Autodesk Inventor part; units mm, degrees
ref_plane "YZ Plane" through (0, 0, 0) normal (1, 0, 0) x (0, 1, 0)
ref_plane "XZ Plane" through (0, 0, 0) normal (0, 1, 0) x (-1, 0, 0)
ref_plane "XY Plane" through (0, 0, 0) normal (0, 0, 1) x (1, 0, 0)
sketch "Sketch_1" plane through (0, 0, 0) normal (0, 0, 1) x (1, 0, 0)
  line L0 (23, 0) -> (0, 0)
  line L1 (0, 0) -> (0, 4.5)
  line L2 (0, 4.5) -> (0.5, 5)
  line L3 (0.5, 5) -> (22.5, 5)
  line L4 (22.5, 5) -> (23, 4.5)
  line L5 (23, 4.5) -> (23, 0)
  line L6 (23, 0) -> (0, 0)
revolve "Revolution1" add sketch "Sketch_1" angle 360 about axis through (23, 0, 0) along (1, 0, 0)
sketch "Sketch2" plane through (0, 0, 0) normal (-1, 0, 0) x (0, 0, 1)
  point P0 (0, 0)
hole "Hole1" at (0, 0, 0) direction (1, 0, 0) diameter 4.134 depth 15.3066 tip angle 120 countersink diameter 5 countersink angle 90
sketch "Sketch_8" plane through (0, 0, 0) normal (0, 0, 1) x (1, 0, 0)
  line L0 (23, 0) -> (-23, 0)
  line L1 (20, 14.8) -> (20, 4.8)
  line L2 (20, 4.8) -> (21.15, 4.8)
  line L3 (21.15, 4.8) -> (21.15, 14.8)
  line L4 (21.15, 14.8) -> (20, 14.8)
revolve "Revolution2" cut sketch "Sketch_8" angle 360 about axis through (23, 0, 0) along (1, 0, 0)
properties part number "FSSFJBF-D10-L20-M5-U3"
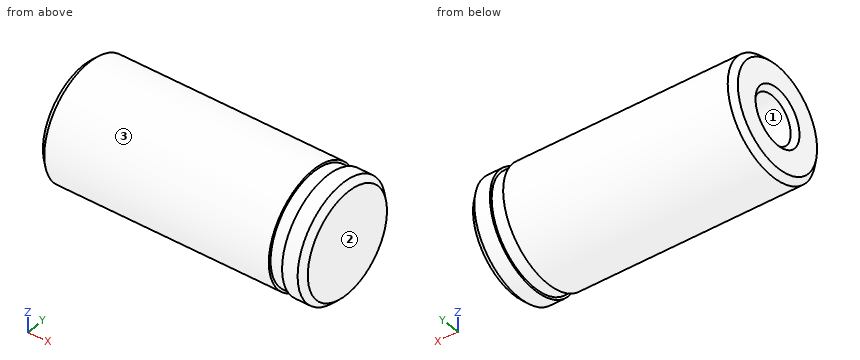
The listing builds one solid part. Answer for the finished solid, in the listing's coordinates (mm). Face numbers are marked on the shaded views. Coordinates: 2 decimals unless noted, no trailing zeros. Loops run counter-clockwise (first coordinate to the right, second up) from the corner with the lowest first, then second, coordinate; pieces in that order, holes last. Notation, with made-up numbers: (23, 61) -> (76, 61) arc R21 cw to (76, 66) -> close; hole circle Ø11 at (54, -18). An arc over 180 degrees is marked (long way). Answer in a Markdown table with one row per item. Add a question column.
1. The part is cut by section A-A, the plane x = 4. Write down the section's boundary in (y, z).
2. Determine the mould class of the marked faces 1, 2 and 3 for opening direction Y: +Y half, -Y half, draft (parallel to the pull), parting line (faces both ways), or undercut.
3. Consider line 1 (Z direction, x = 7.5, y = 0); line 2 (Z direction, x = 9.75, y = -0.5); line 3 (Y direction, x = 13.75, z = -1.5). Determine where each line is inside the solid, lowest interval first. Write a range as [from, to].
4. The part is cut by section B-B, the plane x = 19. Write down the section's boundary in (y, z).
5. Flat-ended cylindrical pins translate along their axes: P1, Ø4, axis at x = 9.5, y = -4, coming from the +Z side; P2, Ø3, axis at x = 19.5, z = 2, coming from the -Y side. Find the tip coordinate at first contact, or state that the pin passes through.
Answer below:
| question | item | result |
|---|---|---|
| 1 | outline | circle Ø10 at (0, 0); hole circle Ø4.13 at (0, 0) |
| 2 | face 1 | undercut |
| 2 | face 2 | draft |
| 2 | face 3 | parting line |
| 3 | line 1 | [-5, -2.07], [2.07, 5] |
| 3 | line 2 | [-4.97, -2.01], [2.01, 4.97] |
| 3 | line 3 | [-4.77, -1.42], [1.42, 4.77] |
| 4 | outline | circle Ø10 at (0, 0) |
| 5 | P1 | z = 4.58 |
| 5 | P2 | y = -4.97 |
